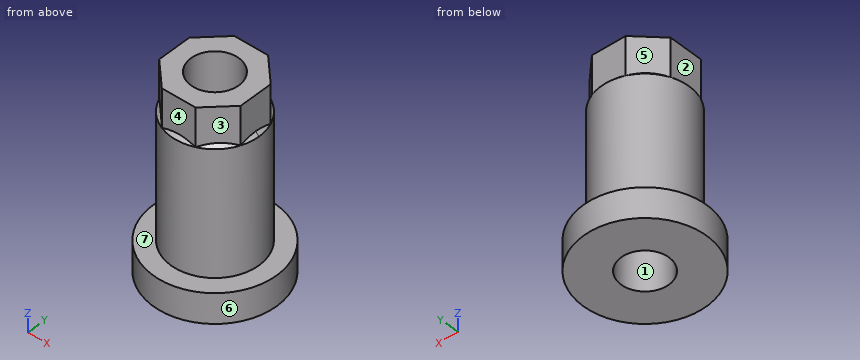
```python
from build123d import *

# Parameters (mm, degrees)
F0_R         = 5.55625
F0_R_2       = 2.15265
F1_DEPTH     = 2.69875
F2_R         = 3.96875
F2_R_2       = 2.15265
F3_DEPTH     = 11.58875
F4_R         = 2.15265
F5_DEPTH     = 3.175
F6_T4_ANGLE  = 45
F6_T9_ANGLE  = 45
F6_T14_ANGLE = 45
F6_T19_ANGLE = 45
F6_T24_ANGLE = 45
F6_T29_ANGLE = 45
F6_T34_ANGLE = 45
F6_T39_ANGLE = 22.5
F6_T44_ANGLE = 22.5


# Not quite as in the source:
# - a fillet or chamfer that OpenCascade refuses, or shapes differently, is made with other operations: its cross-section is extruded or revolved along the edge and cut away or added


with BuildPart() as f1:
    # F0 (on Top) → F1 (new body)
    with BuildSketch(Plane.XY):
        Circle(F0_R)
        Circle(F0_R_2, mode=Mode.SUBTRACT)
    extrude(amount=F1_DEPTH)

    # F2 (on face) → F3 (join)
    with BuildSketch(Plane.XY.offset(2.69875)):
        Circle(F2_R)
        Circle(F2_R_2, mode=Mode.SUBTRACT)
    extrude(amount=F3_DEPTH)

    # F4 (on face) → F5 (join)
    with BuildSketch(Plane.XY.offset(14.2875)):
        Polygon((-3.6666468947, 1.5187748722), (-3.6666468947, -1.5187748722), (-1.5187748722, -3.6666468947), (1.5187748722, -3.6666468947), (3.6666468947, -1.5187748722), (3.6666468947, 1.5187748722), (1.5187748722, 3.6666468947), (-1.5187748722, 3.6666468947), align=None)
        Circle(F4_R, mode=Mode.SUBTRACT)
    extrude(amount=F5_DEPTH)

    # F6: chamfer of 0.3021076 on 7 edges, made by hand


with BuildPart() as f6_tool2:
    # F6_s3 → F6_t4 (revolve)
    with BuildSketch(Plane(origin=(0, 0, 0), x_dir=(0, 0, 1), z_dir=(0.3826834324, 0.9238795325, 0))):
        Polygon((13.9853924, -3.96875), (14.2875, -3.6666424), (14.2875, -3.96875), align=None)
    revolve(axis=Axis((0, 0, 14.2875), (0, 0, 1)), revolution_arc=F6_T4_ANGLE)

    split(bisect_by=Plane.YZ.offset(-3.6666468947), keep=Keep.BOTTOM)


with BuildPart() as f1_1:
    add(f1.part)

    # F6_t1: cut F6_tool2
    add(f6_tool2.part, mode=Mode.SUBTRACT)


with BuildPart() as f6_tool7:
    # F6_s8 → F6_t9 (revolve)
    with BuildSketch(Plane(origin=(0, 0, 0), x_dir=(0, 0, 1), z_dir=(0.9238795325, 0.3826834324, 0))):
        Polygon((13.9853924, -3.96875), (14.2875, -3.6666424), (14.2875, -3.96875), align=None)
    revolve(axis=Axis((0, 0, 14.2875), (0, 0, 1)), revolution_arc=F6_T9_ANGLE)

    split(bisect_by=Plane(origin=(-2.5927108834, 2.5927108834, 0), x_dir=(0, 0, 1), z_dir=(-0.7071067812, 0.7071067812, 0)), keep=Keep.TOP)


with BuildPart() as f1_2:
    add(f1_1.part)

    # F6_t6: cut F6_tool7
    add(f6_tool7.part, mode=Mode.SUBTRACT)


with BuildPart() as f6_tool12:
    # F6_s13 → F6_t14 (revolve)
    with BuildSketch(Plane(origin=(0, 0, 0), x_dir=(0, 0, 1), z_dir=(0.9238795325, -0.3826834324, 0))):
        Polygon((13.9853924, -3.96875), (14.2875, -3.6666424), (14.2875, -3.96875), align=None)
    revolve(axis=Axis((0, 0, 14.2875), (0, 0, 1)), revolution_arc=F6_T14_ANGLE)

    split(bisect_by=Plane.XZ.offset(-3.6666468947), keep=Keep.BOTTOM)


with BuildPart() as f1_3:
    add(f1_2.part)

    # F6_t11: cut F6_tool12
    add(f6_tool12.part, mode=Mode.SUBTRACT)


with BuildPart() as f6_tool17:
    # F6_s18 → F6_t19 (revolve)
    with BuildSketch(Plane(origin=(0, 0, 0), x_dir=(0, 0, 1), z_dir=(0.3826834324, -0.9238795325, 0))):
        Polygon((13.9853924, -3.96875), (14.2875, -3.6666424), (14.2875, -3.96875), align=None)
    revolve(axis=Axis((0, 0, 14.2875), (0, 0, 1)), revolution_arc=F6_T19_ANGLE)

    split(bisect_by=Plane(origin=(2.5927108834, 2.5927108834, 0), x_dir=(0, 0, 1), z_dir=(0.7071067812, 0.7071067812, 0)), keep=Keep.TOP)


with BuildPart() as f1_4:
    add(f1_3.part)

    # F6_t16: cut F6_tool17
    add(f6_tool17.part, mode=Mode.SUBTRACT)


with BuildPart() as f6_tool22:
    # F6_s23 → F6_t24 (revolve)
    with BuildSketch(Plane(origin=(0, 0, 0), x_dir=(0, 0, 1), z_dir=(-0.9238795325, -0.3826834324, 0))):
        Polygon((13.9853924, -3.96875), (14.2875, -3.6666424), (14.2875, -3.96875), align=None)
    revolve(axis=Axis((0, 0, 14.2875), (0, 0, 1)), revolution_arc=F6_T24_ANGLE)

    split(bisect_by=Plane(origin=(2.5927108834, -2.5927108834, 0), x_dir=(0, 0, 1), z_dir=(0.7071067812, -0.7071067812, 0)), keep=Keep.TOP)


with BuildPart() as f1_5:
    add(f1_4.part)

    # F6_t21: cut F6_tool22
    add(f6_tool22.part, mode=Mode.SUBTRACT)


with BuildPart() as f6_tool27:
    # F6_s28 → F6_t29 (revolve)
    with BuildSketch(Plane(origin=(0, 0, 0), x_dir=(0, 0, 1), z_dir=(-0.9238795325, 0.3826834324, 0))):
        Polygon((13.9853924, -3.96875), (14.2875, -3.6666424), (14.2875, -3.96875), align=None)
    revolve(axis=Axis((0, 0, 14.2875), (0, 0, 1)), revolution_arc=F6_T29_ANGLE)

    split(bisect_by=Plane.XZ.offset(3.6666468947), keep=Keep.TOP)


with BuildPart() as f1_6:
    add(f1_5.part)

    # F6_t26: cut F6_tool27
    add(f6_tool27.part, mode=Mode.SUBTRACT)


with BuildPart() as f6_tool32:
    # F6_s33 → F6_t34 (revolve)
    with BuildSketch(Plane(origin=(0, 0, 0), x_dir=(0, 0, 1), z_dir=(-0.3826834324, 0.9238795325, 0))):
        Polygon((13.9853924, -3.96875), (14.2875, -3.6666424), (14.2875, -3.96875), align=None)
    revolve(axis=Axis((0, 0, 14.2875), (0, 0, 1)), revolution_arc=F6_T34_ANGLE)

    split(bisect_by=Plane(origin=(-2.5927108834, -2.5927108834, 0), x_dir=(0, 0, 1), z_dir=(-0.7071067812, -0.7071067812, 0)), keep=Keep.TOP)


with BuildPart() as f1_7:
    add(f1_6.part)

    # F6_t31: cut F6_tool32
    add(f6_tool32.part, mode=Mode.SUBTRACT)


with BuildPart() as f6_tool37:
    # F6_s38 → F6_t39 (revolve)
    with BuildSketch(Plane(origin=(0, 0, 0), x_dir=(0, 0, 1), z_dir=(-0.3826834324, -0.9238795325, 0))):
        Polygon((13.9853924, -3.96875), (14.2875, -3.6666424), (14.2875, -3.96875), align=None)
    revolve(axis=Axis((0, 0, 14.2875), (0, 0, 1)), revolution_arc=F6_T39_ANGLE)

    split(bisect_by=Plane.YZ.offset(3.6666468947), keep=Keep.TOP)


with BuildPart() as f1_8:
    add(f1_7.part)

    # F6_t36: cut F6_tool37
    add(f6_tool37.part, mode=Mode.SUBTRACT)


with BuildPart() as f6_tool42:
    # F6_s43 → F6_t44 (revolve)
    with BuildSketch(Plane.XZ):
        Polygon((3.96875, 13.9853924), (3.6666424, 14.2875), (3.96875, 14.2875), align=None)
    revolve(axis=Axis((0, 0, 14.2875), (0, 0, 1)), revolution_arc=F6_T44_ANGLE)

    split(bisect_by=Plane.YZ.offset(3.6666468947), keep=Keep.TOP)


with BuildPart() as f1_9:
    add(f1_8.part)

    # F6_t41: cut F6_tool42
    add(f6_tool42.part, mode=Mode.SUBTRACT)


solid = f1_9.part
```
Verification items for the finished model (mm, model axes). Face numbers are marked on the shaded views. A direction names the side the tool comes from. Coordinates: 2 decimals unless noted, no trailing zeros. Loops run counter-clockwise (first coordinate to the right, second up) from the corner with the lowest first, then second, coordinate; pieces in that order, holes last. Notation, with made-up numbers: (63.25, 16.25) - (82.25, 16.25) arc R15 cw to (82.25, 31.25) - close; hole circle Ø9 at (86.25, -7). An arc over 180 degrees is marked (long way). Put each result on its own line as item: value.
Item 1: Section check D-D (y = 5). Enter the section's corners in (x, z).
Conclusion:
outline: (-2.42, 0) - (2.42, 0) - (2.42, 2.7) - (-2.42, 2.7) - close
Item 2: Section check A-A (x = 0). Enter the section's corners in (y, z).
Conclusion:
outline: (-5.56, 0) - (-2.15, 0) - (-2.15, 17.46) - (-3.67, 17.46) - (-3.67, 14.29) - (-3.97, 13.99) - (-3.97, 2.7) - (-5.56, 2.7) - close; (2.15, 0) - (5.56, 0) - (5.56, 2.7) - (3.97, 2.7) - (3.97, 13.99) - (3.67, 14.29) - (3.67, 17.46) - (2.15, 17.46) - close
Item 3: Gauge pin test, flat ends, axial feed: pin 1 Ø3.5 at (y, z) = (-0.5, 16.5) entering from -X; pin 2 Ø4 at (y, z) = (0.5, 8) entering from -X; pin 3 Ø3 at (x, z) = (-2.5, 4) entering from -Y; pin 4 Ø5 at (x, y) = (0.5, 4) entering from -Z. Record the tip position at first contact, or that the pin passes through.
Conclusion:
pin 1: stops at x = -3.67
pin 2: stops at x = -3.97
pin 3: stops at y = -5.27
pin 4: stops at z = 0
Item 4: Section check C-C (y = -4.5). Enter the section's corners in (x, z).
Conclusion:
outline: (-3.26, 0) - (3.26, 0) - (3.26, 2.7) - (-3.26, 2.7) - close
Item 5: Scan lines: line 1 along Y through (x, z) = (0, 13); line 2 along Y through (x, z) = (0, 1); line 3 along Z through (x, y) = (-1.5, -4). Record each from-to range of solid material in increasing order.
Conclusion:
line 1: y = -3.97 to -2.15, 2.15 to 3.97
line 2: y = -5.56 to -2.15, 2.15 to 5.56
line 3: z = 0 to 2.7
Item 6: Set-up check for the marked faces 5, 6 and 7: record each of +Z, -Z, +X, -X, +Y, -Y from which the full face is reachable in a straight line by a thin tool's end or side.
Conclusion:
face 5: +Z, -X, +Y
face 6: +Z, -Z
face 7: +Z
Item 7: Draft check along X on the marked faces 1, 2, 3 and 4. Enter one of: pulls with the +X half, pulls with the -X half, needs draft (parallel to the pull), parting line crosses it, or undercut.
Conclusion:
face 1: undercut
face 2: pulls with the -X half
face 3: pulls with the +X half
face 4: needs draft
Item 8: Section check B-B (z = 4.25). Enter the section's corners in (x, y), then the cut area to 3 significant figures.
Conclusion:
outline: circle Ø7.94 at (0, 0); hole circle Ø4.31 at (0, 0)
area: 34.9 mm2
